Geometry: final body of the model. Coordinates: model frame, mm. A direction names the side the tool comes from. Give positions to 0.01 mm unless a question says otherwise; leave off trailing zeros. Write each loop counter-clockwise with the first axis right and the second up, starting at its lowest first coordinate (ties: lowest second). Pieces come first, ordered by that corner, then holes. Notation, with made-up numbers: (82, 40) -> (111, 40) arc R30 cw to (111, 68) -> close; hole circle Ø7 at (39, 42). An arc over 180 degrees is marked (long way). Answer in a Markdown table with one row per item. Add a question column.
Item 1: Section query D-D on x = 941. Output: boundary loops of the cut face in (y, z), plus the area to 3 significant figures.
Item 2: Draft query along X for faces 1 (the flat face through (777.623, -19, 542)), 2 (the flat face through (834, -660.4, 1075)), 3 (the flat face through (688.723, -19, 618)). Return one class per face: +X half, -X half, draft (parallel to the pull), parting line (faces both ways), or undercut.
Item 3: Material intervals for probe 1 along Y at (x, z) = (731, 308); probe 2 along X at (y, z) = (-75, 664.5); probe 3 along X at (y, z) = (-473, 165), sorted ascending. Write a range as from..to.
Item 4: First-contact query: P1, Ø23, axis at x = 839.5, z = 1056.5, coming from the -Y side; P2, Ø6, axis at x = 910.5, y = -1095.5, coming from the -Z side; P3, Ø1.5, axis at x = 1295, y = -231.5, coming from the +Z side. Flat tips, straight axial feed; report the tip coordinate or a pass-through.
Item 5: Access query for faces 4 (the flat face through (733, -38.1, 618)), 5 (the flat face through (835, -152.4, 1074)), 6 (the flat face through (834, -254, 1075)), 7 (the flat face through (777.623, -1200, 542)). Directions: +Z, -Z, +X, -X, +Y, -Y. A direction counts if a zero-diameter tool reaches every point of the face in a straight line with its end or side. Return the directions, or none.
Item 6: Section query A-A on y = -223.5. Output: boundary loops of the cut face in (x, z), plus the area to 3 significant figures.
Item 7: Section query C-C on y = -370. Output: boundary loops of the cut face in (x, z), plus the area to 3 significant figures.
Item 8: Section query B-B on z = 851. Output: boundary loops of the cut face in (x, y).
```python
from build123d import *

# Parameters (mm, degrees)
F1_DEPTH = 1219.2
F2_DEPTH = 1219.2
F3_W     = 88.9
F3_H     = 38.1
F6_W     = 101.6
F6_H     = 44.45
F6_W_2   = 50.8
F7_DEPTH = 38.1


# Not quite as in the source:
# - a feature of the source that left no trace in its solid (it failed there, or was rolled back) is left out


with BuildPart() as f1:
    # F0 (on Front) → F1 (new body)
    with BuildSketch(Plane.XZ):
        Polygon((1412.622521745, 0), (1428.0204534243, 8.89), (818.4204534243, 1064.748172294), (803.022521745, 1055.858172294), align=None)
    extrude(amount=F1_DEPTH)

    # F0 (on Front) → F2 (join, through all)
    with BuildSketch(Plane.XZ):
        Polygon((803.022521745, 1055.858172294), (818.4204534243, 1064.748172294), (513.6204534243, 1592.677258441), (498.222521745, 1583.787258441), align=None)
    extrude(amount=F2_DEPTH)

    # F3 (on Top) → F5 (join, up to the next surface of F1)
    with BuildSketch(Plane.XY):
        with Locations((733.172521745, -19.05)):
            Rectangle(F3_W, F3_H)
        with Locations((733.172521745, -1200.15)):
            Rectangle(F3_W, F3_H)
    extrude(until=Until.NEXT)

    # F6 (on face) → F7 (join)
    with BuildSketch(Plane(origin=(1074.864822988, 0, 620.5734948946), x_dir=(0, 1, 0), z_dir=(0.8660254038, 0, 0.5))):
        with Locations((-203.2, 490.6637391275)):
            Rectangle(F6_W, F6_H)
        with Locations((-203.2, 535.1137391275)):
            Rectangle(F6_W, F6_H)
        with Locations((-1016, 490.6637391275)):
            Rectangle(F6_W, F6_H)
        with Locations((-1016, 535.1137391275)):
            Rectangle(F6_W, F6_H)
        Polygon((-558.8, 468.4387391275), (-558.8, 512.8887391275), (-609.6, 512.8887391275), (-660.4, 512.8887391275), (-660.4, 468.4387391275), align=None)
        with Locations((-584.2, 535.1137391275)):
            Rectangle(F6_W_2, F6_H)
        with Locations((-635, 535.1137391275)):
            Rectangle(F6_W_2, F6_H)
    extrude(amount=F7_DEPTH)


solid = f1.part
```
Findings below:
| question | item | result |
|---|---|---|
| 1 | outline | (-1219.2, 816.87) -> (0, 816.87) -> (0, 852.43) -> (-1219.2, 852.43) -> close |
| 1 | area | 43,400 mm^2 |
| 2 | face 1 | undercut |
| 2 | face 2 | draft |
| 2 | face 3 | -X half |
| 3 | probe 1 | y = -1219.2..-1181.1, -38.1..0 |
| 3 | probe 2 | x = 1028.97..1049.5 |
| 3 | probe 3 | x = 1317.36..1337.89 |
| 4 | P1 | stops at y = -1066.8 |
| 4 | P2 | stops at z = 864.51 |
| 4 | P3 | stops at z = 240.59 |
| 5 | face 4 | -Z, -X |
| 5 | face 5 | +Z, +X, +Y |
| 5 | face 6 | +Z, +X |
| 5 | face 7 | -Z, +Y, -Y |
| 6 | outline | (498.22, 1583.79) -> (1412.62, 0) -> (1428.02, 8.89) -> (840.65, 1026.25) -> (873.64, 1045.3) -> (829.19, 1122.29) -> (796.2, 1103.24) -> (513.62, 1592.68) -> close |
| 6 | area | 35,900 mm^2 |
| 7 | outline | (498.22, 1583.79) -> (1412.62, 0) -> (1428.02, 8.89) -> (513.62, 1592.68) -> close |
| 7 | area | 32,500 mm^2 |
| 8 | outline | (688.72, -1219.2) -> (777.62, -1219.2) -> (777.62, -1181.1) -> (688.72, -1181.1) -> close; (688.72, -38.1) -> (777.62, -38.1) -> (777.62, 0) -> (688.72, 0) -> close; (921.3, -1219.2) -> (941.83, -1219.2) -> (941.83, 0) -> (921.3, 0) -> close |
